Design review of the part built by this model. Coordinates are the model's own, in mm. Face numbers are marked on the shaded views. A direction names the side the tool comes from. Round coordinates to 2 decimals unless told otherwise and drop trailing zeros. Order: outer loops, then holes, each group sorted by start corner. A loop starts at its lowest first (then second) coordinate and runs counter-clockwise, first axis right, second up. Notation, with made-up numbers: (31, -32.75) - (69, -32.75) arc R17 ccw to (69, -26.75) - close; hole circle Ø1 at (85, -13). An arc over 180 degrees is marked (long way). Write item = value, one per line.
Autodesk Inventor part; units mm, degrees
ref_plane "YZ Plane" through (0, 0, 0) normal (1, 0, 0) x (0, 1, 0)
ref_plane "XZ Plane" through (0, 0, 0) normal (0, 1, 0) x (-1, 0, 0)
ref_plane "XY Plane" through (0, 0, 0) normal (0, 0, 1) x (1, 0, 0)
sketch "스케치1" plane through (0, 0, 0) normal (0, 0, 1) x (1, 0, 0)
  arc A0 (-10, 0) -> (0, -10) centre (0, 0) ccw
  line L0 (-30.8853, 0) -> (100.8142, 0)
  line L1 (0, -14.9853) -> (0, 5.4142)
  line L2 (-10, 0) -> (-10, 2.5)
  line L3 (-10, 2.5) -> (0, 2.5)
  dimension "d1" = 20
  dimension "d2" = 2.5
sketch "스케치2" plane through (0, 0, 0) normal (0, 0, 1) x (1, 0, 0)
  line L0 (0, -14.9853) -> (0, 5.4142)
  line L1 (-30.8853, 0) -> (100.8142, 0)
  line L2 (-10, 2.5) -> (0, 2.5)
  line L3 (0, 2.5) -> (0, -9)
  line L4 (0, -9) -> (18, -9)
  line L5 (18, -9) -> (18, 2.5)
  line L6 (18, 2.5) -> (20, 2.5)
  line L7 (20, 2.5) -> (20, -9)
  line L8 (20, -9) -> (48, -9)
  line L9 (48, -9) -> (48, 2.5)
  line L10 (48, 2.5) -> (50, 2.5)
  line L11 (50, 2.5) -> (50, -9)
  line L12 (50, -9) -> (78, -9)
  line L13 (78, -9) -> (78, 2.5)
  line L14 (78, 2.5) -> (82, 2.5)
  line L15 (82, 2.5) -> (82, -9)
  line L16 (82, -9) -> (82, -10)
  line L17 (0, -10) -> (82, -10)
  point P0 (0, 0)
  dimension "d3" = 11.5
  dimension "d4" = 18
  dimension "d5" = 2
  dimension "d6" = 11.5
  dimension "d7" = 28
  dimension "d8" = 2
  dimension "d9" = 11.5
  dimension "d10" = 28
  dimension "d11" = 4
  dimension "d12" = 11.5
  dimension "d13" = 1
sketch "스케치3" plane through (0, 0, 0) normal (0, 0, 1) x (1, 0, 0)
  arc A0 (-10, 0) -> (0, -10) centre (0, 0) ccw
  line L0 (-10, 0) -> (-10, 2.5)
  line L1 (-10, 2.5) -> (0, 2.5)
  line L2 (0, -9) -> (18, -9)
  line L3 (0, -10) -> (82, -10)
  line L4 (18, -9) -> (18, 2.5)
  line L5 (18, 2.5) -> (20, 2.5)
  line L6 (20, 2.5) -> (20, -9)
  line L7 (20, -9) -> (48, -9)
  line L8 (48, -9) -> (48, 2.5)
  line L9 (50, 2.5) -> (50, -9)
  line L10 (48, 2.5) -> (50, 2.5)
  line L11 (50, -9) -> (78, -9)
  line L12 (78, -9) -> (78, 2.5)
  line L13 (78, 2.5) -> (82, 2.5)
  line L14 (82, 2.5) -> (82, -9)
extrude "돌출1" add sketch "스케치2" along normal blind 24 contours L0 L4 L5 L1 L7 L8 L9 L11 L12 L13 L15 L16 L17 | L5 L6 L7 L1 | L1 L13 L14 L15 | L9 L10 L11 L1
extrude "돌출2" add sketch "스케치1" along normal blind 24
sketch "스케치4" plane through (0, -9, 0) normal (1, 0, 0) x (0, 0, -1)
  point P0 (0, 9)
sketch "스케치5" plane through (0, -9, 0) normal (1, 0, 0) x (0, 0, -1)
  line L0 (-6.205, 11.5) -> (-6.205, 9.9472)
  line L1 (-6.205, 9.9472) -> (-7.7578, 7.2578)
  line L2 (-7.7578, 7.2578) -> (-10.4472, 5.705)
  line L3 (-10.4472, 5.705) -> (-13.5528, 5.705)
  line L4 (-13.5528, 5.705) -> (-16.2422, 7.2578)
  line L5 (-16.2422, 7.2578) -> (-17.795, 9.9472)
  line L6 (-17.795, 9.9472) -> (-17.795, 11.5)
  line L7 (0, 0) -> (-24, 0)
  line L8 (0, 11.5) -> (-24, 11.5)
  point P0 (0, 9)
  point P1 (-12, 11.5)
  point P2 (-12, 0)
  point P3 (-12, 11.5)
  dimension "d18" = 11.59
extrude "돌출3" cut sketch "스케치5" against normal blind 4
sketch "스케치6" plane through (0, -9, 0) normal (1, 0, 0) x (0, 0, -1)
  line L0 (-13.5528, 5.705) -> (-16.2422, 7.2578)
  line L1 (-10.4472, 5.705) -> (-13.5528, 5.705)
  line L2 (-7.7578, 7.2578) -> (-10.4472, 5.705)
  line L3 (-6.205, 9.9472) -> (-7.7578, 7.2578)
  line L4 (-6.205, 11.5) -> (-6.205, 9.9472)
  line L5 (-17.795, 11.5) -> (-6.205, 11.5)
  line L6 (-17.795, 9.9472) -> (-17.795, 11.5)
  line L7 (-16.2422, 7.2578) -> (-17.795, 9.9472)
  point P0 (0, 9)
extrude "돌출4" cut sketch "스케치6" along normal blind 80
sketch "스케치7" plane through (82, -10, 0) normal (1, 0, 0) x (0, 0, -1)
  point P0 (0, 10)
sketch "스케치8" plane through (80, -9, 0) normal (-1, 0, 0) x (0, 0, 1)
  line L0 (6.205, 11.5) -> (17.795, 11.5)
  line L1 (10.4472, 5.705) -> (7.7578, 7.2578)
  line L2 (13.5528, 5.705) -> (10.4472, 5.705)
  line L3 (16.2422, 7.2578) -> (13.5528, 5.705)
  line L4 (17.795, 9.9472) -> (16.2422, 7.2578)
  line L5 (17.795, 11.5) -> (17.795, 9.9472)
  line L6 (6.205, 11.5) -> (17.795, 11.5)
  line L7 (6.205, 9.9472) -> (6.205, 11.5)
  line L8 (7.7578, 7.2578) -> (6.205, 9.9472)
  point P0 (0, 9)
sketch "스케치9" plane through (82, -10, 0) normal (1, 0, 0) x (0, 0, -1)
  arc A0 (-15.055, 12.5) -> (-8.945, 12.5) centre (-12, 12.5) ccw
  line L0 (0, 12.5) -> (-24, 12.5)
  point P0 (0, 10)
extrude "돌출5" cut sketch "스케치9" against normal up to surface (2 mm away)
properties part number "Support"
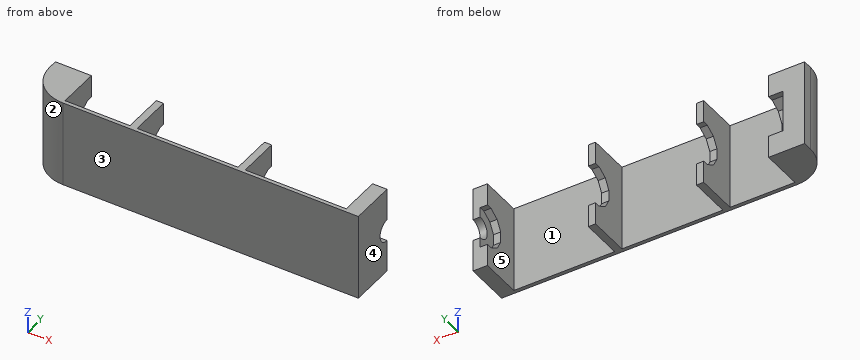
Item 1: Take a section at A-A, the plane z = 12. State the section outline as (x, y) points (3 decimals), and give its area (3 significant figures).
Data:
outline = (-10, 0) arc R10 ccw to (0, -10) - (82, -10) - (82, -0.555) - (80, -0.555) - (80, -3.295) - (78, -3.295) - (78, -9) - (50, -9) - (50, -3.295) - (48, -3.295) - (48, -9) - (20, -9) - (20, -3.295) - (18, -3.295) - (18, -9) - (0, -9) - (0, -3.295) - (-4, -3.295) - (-4, 2.5) - (-10, 2.5) - close
area = 213 mm2
Item 2: For line 1 along X through (y, z) = (0, 5); line 2 along X through (y, z) = (-2.5, 4); line 3 along X through (y, z) = (-0.25, 7.75), list the stretches that pass through material, from the lowest coordinate up. Write a range as [from, to].
Data:
line_1 = [-10, 0], [18, 20], [48, 50], [78, 82]
line_2 = [-9.68, 0], [18, 20], [48, 50], [78, 82]
line_3 = [-10, -4], [80, 82]
Item 3: Take a section at B-B, the plane y = -5.5. State the section outline as (x, z) points, and give its area (3 significant figures).
Data:
outline = (-8.35, 0) - (0, 0) - (0, 24) - (-8.35, 24) - close; (18, 0) - (20, 0) - (20, 24) - (18, 24) - close; (48, 0) - (50, 0) - (50, 24) - (48, 24) - close; (78, 0) - (82, 0) - (82, 24) - (78, 24) - close
area = 392 mm2
Item 4: The part is to be moulded in two halves that separate along X. For the marked faces 1, 2 and 3, say which applies: +X half, -X half, draft (parallel to the pull), parting line (faces both ways), or undercut.
Data:
face_1 = undercut
face_2 = -X half
face_3 = draft
Item 5: Take a section at D-D, the plane z = 19. State the section outline as (x, y) points.
Data:
outline = (-10, 0) arc R10 ccw to (0, -10) - (82, -10) - (82, 2.5) - (78, 2.5) - (78, -9) - (50, -9) - (50, 2.5) - (48, 2.5) - (48, -9) - (20, -9) - (20, 2.5) - (18, 2.5) - (18, -9) - (0, -9) - (0, 2.5) - (-10, 2.5) - close
Item 6: For the marked faces 4 and 5, list the 3-axis set-ups (+Z, -Z, +X, -X, +Y, -Y) from which the entire face can be reached by the end or side of a thin tool; tool diameter is ignored.
Data:
face_4 = +Z, -Z, +X, +Y, -Y
face_5 = +Z, -Z, +Y
Item 7: Insertion check: P1, Ø1.5, axis at x = 69.5, y = -8, coming from the -Z side; P2, Ø0.6, axis at x = 19, z = 12, coming from the +Y side (3 decimals); P3, Ø1.6, axis at x = 79.5, z = 11.5, coming from the +Y side; P4, Ø6, axis at y = -5, z = 17, coming from the -X side. Each pin has a flat end and moves straight along its axis. Give the tip position at first contact, or say it passes through.
Data:
P1 = through
P2 = -3.295
P3 = -0.34
P4 = -9.8
Item 8: Take a section at C-C, the plane x = 40.5. State the section outline as (y, z) points, and give its area (3 significant figures).
Data:
outline = (-10, 0) - (-9, 0) - (-9, 24) - (-10, 24) - close
area = 24.0 mm2
